from build123d import *

# Parameters (mm, degrees)
F0_W     = 187
F0_H     = 20
F3_DEPTH = 100
F4_DEPTH = 85


with BuildPart() as f1:
    # F0 (on Front) → F1 (revolve)
    with BuildSketch(Plane.XZ):
        Polygon((47, 28), (47, 0), (60, 0), (60, 42.5), (47, 42.5), align=None)
        with Locations((-93.5, 10)):
            Rectangle(F0_W, F0_H)
        Polygon((0, 20), (0, 0), (47, 0), (47, 28), (0, 28), align=None)
    revolve(axis=Axis((-82.005277276, 0, 0), (-1, 0, 0)))

    # F2 (on Top) → F3 (join)
    with BuildSketch(Plane.XY):
        with BuildLine():
            ThreePointArc((-167.5, 5), (-171.0355339059, 3.5355339059), (-172.5, 0))
            Line((-172.5, 0), (-167.5, 0))
            Line((-167.5, 0), (-162.5, 0))
            ThreePointArc((-162.5, 0), (-163.9644660941, 3.5355339059), (-167.5, 5))
        make_face()
        with BuildLine():
            Line((-167.5, 0), (-172.5, 0))
            ThreePointArc((-172.5, 0), (-171.0355339059, -3.5355339059), (-167.5, -5))
            ThreePointArc((-167.5, -5), (-163.9644660941, -3.5355339059), (-162.5, 0))
            Line((-162.5, 0), (-167.5, 0))
        make_face()
        with BuildLine():
            Line((-137.5, 5), (-167.5, 5))
            ThreePointArc((-167.5, 5), (-163.9644660941, 3.5355339059), (-162.5, 0))
            Line((-162.5, 0), (-142.5, 0))
            ThreePointArc((-142.5, 0), (-141.0355339059, 3.5355339059), (-137.5, 5))
        make_face()
        with BuildLine():
            ThreePointArc((-162.5, 0), (-163.9644660941, -3.5355339059), (-167.5, -5))
            Line((-167.5, -5), (-137.5, -5))
            ThreePointArc((-137.5, -5), (-141.0355339059, -3.5355339059), (-142.5, 0))
            Line((-142.5, 0), (-162.5, 0))
        make_face()
        with BuildLine():
            Line((-137.5, 0), (-137.5, 5))
            ThreePointArc((-137.5, 5), (-141.0355339059, 3.5355339059), (-142.5, 0))
            Line((-142.5, 0), (-137.5, 0))
        make_face()
        with BuildLine():
            ThreePointArc((-132.5, 0), (-133.9644660941, 3.5355339059), (-137.5, 5))
            Line((-137.5, 5), (-137.5, 0))
            Line((-137.5, 0), (-137.5, -5))
            ThreePointArc((-137.5, -5), (-133.9644660941, -3.5355339059), (-132.5, 0))
        make_face()
        with BuildLine():
            ThreePointArc((-142.5, 0), (-141.0355339059, -3.5355339059), (-137.5, -5))
            Line((-137.5, -5), (-137.5, 0))
            Line((-137.5, 0), (-142.5, 0))
        make_face()
    extrude(amount=F3_DEPTH)

    # F4 (cut): a face of the model
    f4_faces = [f1.faces().sort_by_distance(p)[0] for p in [
        (-152.5, 0, 100),
    ]]
    extrude(f4_faces, amount=-F4_DEPTH, mode=Mode.SUBTRACT)


solid = f1.part
Work out the finished part from the listing and answer in its coordinate system (mm). A direction names the side the tool comes from. Coordinates: 2 decimals unless noted, no trailing zeros. Loops run counter-clockwise (first coordinate to the right, second up) from the corner with the lowest first, then second, coordinate; pieces in that order, holes last. Notation, with made-up numbers: (20.25, 59.5) -> (45.25, 59.5) arc R14 cw to (45.25, 72.5) -> close; hole circle Ø3 at (52.5, -28.5). An arc over 180 degrees is marked (long way). Write each question's results on one line, items separated by ' | '. Start each with the question number.
1) Find section D-D on x = 22. Determine the outline of the cut face in (y, z), then the cut area to 3 significant figures.
2) For faces 4 (the flat face through (-187, 0, 0)), 5 (the flat face through (0, 19, -7)), 6 (the flat face through (-153, 0, 15)), determine the directions among +Z, -Z, +X, -X, +Y, -Y from which every point of the face is accessible in a straight line to the end or side of a thin tool.
3) Find section A-A on z = 0. Determine the outline of the cut face in (x, y).
4) Flat-ended cylindrical pins translate along their axes: P1, Ø4, axis at y = 29, z = -1, coming from the -X side; P2, Ø3.5, axis at x = -145.5, z = 16.5, coming from the +Y side; P3, Ø1, axis at x = -60.5, y = 4.5, coming from the +Z side. Find the tip coordinate at first contact, or state that the pin passes through.
5) Find section B-B on x = -43. Determine the outline of the cut face in (y, z).
6) Consider line 1 along X through (y, z) = (21, 22); line 2 along Y through (x, z) = (-165, 1); line 3 along Z through (x, y) = (-28.5, 0.5). Determine where each line is inside the solid, lowest interval first.
7) Find section C-C on y = -11. Determine the outline of the cut face in (x, z), then the cut area to 3 significant figures.
8) The mould has two halves that part along Y. Classify faces 1 (the cylindrical face through (53.409, -25.861, -33.727)), 2 (the flat face through (-152, 5, 17)), 3 (the flat face through (47, -9, 28)): pulls with the +Y half, pulls with the -Y half, needs draft (parallel to the pull), parting line crosses it, or undercut.
Response values:
1) outline: circle Ø56 at (0, 0) | area: 2,460 mm^2
2) face 4: +Z, -Z, -X, +Y, -Y | face 5: -X | face 6: +Z
3) outline: (-187, -20) -> (0, -20) -> (0, -28) -> (47, -28) -> (47, -42.5) -> (60, -42.5) -> (60, 42.5) -> (47, 42.5) -> (47, 28) -> (0, 28) -> (0, 20) -> (-187, 20) -> close
4) P1: stops at x = 0 | P2: stops at y = 13.51 | P3: stops at z = 19.6
5) outline: circle Ø40 at (0, 0)
6) line 1: x = 47 to 60 | line 2: y = -19.97 to 19.97 | line 3: z = -19.99 to 19.99
7) outline: (-187, -16.7) -> (0, -16.7) -> (0, -25.75) -> (47, -25.75) -> (47, -41.05) -> (60, -41.05) -> (60, 41.05) -> (47, 41.05) -> (47, 25.75) -> (0, 25.75) -> (0, 16.7) -> (-187, 16.7) -> close | area: 9,730 mm^2
8) face 1: parting line crosses it | face 2: undercut | face 3: needs draft
